Geometry: final body of the model. Coordinates: model frame, mm. Give positions to 0.01 mm unless a question says otherwise; leave off trailing zeros. Write each loop counter-clockwise with the first axis right and the second up, starting at its lowest first coordinate (ties: lowest second). Pieces come first, ordered by that corner, then holes.
from build123d import *

# Parameters (mm, degrees)
SKIZZE1_W                       = 75
SKIZZE1_H                       = 75
AUFSATZ_LINEAR_AUSTRAGEN1_DEPTH = 3
SKIZZE2_R                       = 14.5
SCHNITT_LINEAR_AUSTRAGEN1_DEPTH = 4
VERRUNDUNG1_R                   = 2
DURCHGANGSLOCH_F_R_M41_D        = 4.5
SCHNITT_LINEAR_AUSTRAGEN2_DEPTH = 4


with BuildPart() as part:
    # Skizze1 → Aufsatz-Linear austragen1 (new body)
    with BuildSketch(Plane.XY):
        Rectangle(SKIZZE1_W, SKIZZE1_H)
    extrude(amount=AUFSATZ_LINEAR_AUSTRAGEN1_DEPTH)

    # Skizze2 → Schnitt-Linear austragen1 (cut, through all)
    with BuildSketch(Plane.XY.offset(3)):
        with Locations((-18, 0)):
            Circle(SKIZZE2_R)
        with Locations((18, 0)):
            Circle(SKIZZE2_R)
    extrude(amount=-SCHNITT_LINEAR_AUSTRAGEN1_DEPTH, mode=Mode.SUBTRACT)

    # Verrundung1
    verrundung1_edges = [part.edges().sort_by_distance(p)[0] for p in [
        (37.5, -37.5, 1.5),
        (-37.5, -37.5, 1.5),
        (-37.5, 37.5, 1.5),
        (37.5, 37.5, 1.5),
    ]]
    fillet(verrundung1_edges, radius=VERRUNDUNG1_R)

    # Durchgangsloch für M41 (through all)
    with Locations(Plane.XY.offset(3)):
        with Locations((27.5, 27.5), (-27.5, 27.5)):
            durchgangsloch_f_r_m41 = Hole(DURCHGANGSLOCH_F_R_M41_D / 2)

    # Spiegeln1: Durchgangsloch für M41 across plane
    add(durchgangsloch_f_r_m41.mirror(Plane.ZX), mode=Mode.SUBTRACT)

    # Skizze6 → Schnitt-Linear austragen2 (cut, through all)
    with BuildSketch(Plane.XY.offset(3)):
        with BuildLine():
            Line((17.791240349, 1.485402103), (33.635529448, 3.712171718))
            ThreePointArc((33.635529448, 3.712171718), (35.329691203, 2.435529267), (34.053048751, 0.741367512))
            Line((34.053048751, 0.741367512), (18.208759651, -1.485402103))
            ThreePointArc((18.208759651, -1.485402103), (16.514597897, -0.208759651), (17.791240349, 1.485402103))
        make_face()
    extrude(amount=-SCHNITT_LINEAR_AUSTRAGEN2_DEPTH, mode=Mode.SUBTRACT)


solid = part.part
Q1. Pin query (flat end, axial travel): P1, Ø3.5, axis at x = 27.5, y = -27.5, coming from the -Z side. Return the tip coordinate at first contact, or that it passes through.
Filled sheet:
P1: passes through
Q2. Section C-C on z = 1.6. Output: boundary loops of the cut face in (x, y), plus the area to 3 significant figures.
Filled sheet:
outline: (-37.5, -35.5) arc R2 ccw to (-35.5, -37.5) - (35.5, -37.5) arc R2 ccw to (37.5, -35.5) - (37.5, 35.5) arc R2 ccw to (35.5, 37.5) - (-35.5, 37.5) arc R2 ccw to (-37.5, 35.5) - close; hole circle Ø29 at (-18, 0); hole circle Ø4.5 at (-27.5, -27.5); hole circle Ø4.5 at (-27.5, 27.5); hole circle Ø4.5 at (27.5, -27.5); hole circle Ø4.5 at (27.5, 27.5); hole (32.07, 3.49) arc R14.5 ccw (long way) to (32.49, 0.52) - (34.05, 0.74) arc R1.5 ccw to (33.64, 3.71) - close
area: 4,230 mm2
Q3. Section B-B on y = 27.5. Output: boundary loops of the cut face in (x, z).
Filled sheet:
outline: (-37.5, 0) - (-29.75, 0) - (-29.75, 3) - (-37.5, 3) - close; (-25.25, 0) - (25.25, 0) - (25.25, 3) - (-25.25, 3) - close; (29.75, 0) - (37.5, 0) - (37.5, 3) - (29.75, 3) - close
Q4. Pull-direction query (Y, two-part tool) for faces 1 (the flat face through (-1, 1, 0)), 2 (the cylindrical face through (-28.538, 25.504, 1.479)), 3 (the cylindrical face through (-36.93, 36.9, 1.52)); classes: released by +Y, released by -Y, zero draft, split by the parting line, or undercut.
Filled sheet:
face 1: zero draft
face 2: undercut
face 3: released by +Y
Q5. Ray query, line 1 along X through (y, z) = (1, 1.85); line 2 along Y through (x, z) = (26.5, 1.8); line 3 along Y through (x, z) = (-26, 2.3). Return the intervals inside material, ascending.
Filled sheet:
line 1: x = -37.5 to -32.47, -3.53 to 3.53, 34.71 to 37.5
line 2: y = -37.5 to -29.52, -25.48 to -11.75, 11.75 to 25.48, 29.52 to 37.5
line 3: y = -37.5 to -29.18, -25.82 to -12.09, 12.09 to 25.82, 29.18 to 37.5
Q6. Section D-D on x = 26.5. Output: boundary loops of the cut face in (y, z), plus the area to 3 significant figures.
Filled sheet:
outline: (-37.5, 0) - (-29.52, 0) - (-29.52, 3) - (-37.5, 3) - close; (-25.48, 0) - (-11.75, 0) - (-11.75, 3) - (-25.48, 3) - close; (11.75, 0) - (25.48, 0) - (25.48, 3) - (11.75, 3) - close; (29.52, 0) - (37.5, 0) - (37.5, 3) - (29.52, 3) - close
area: 130 mm2
Q7. Section A-A on x = -18. Output: boundary loops of the cut face in (y, z), plus the area to 3 significant figures.
Filled sheet:
outline: (-37.5, 0) - (-14.5, 0) - (-14.5, 3) - (-37.5, 3) - close; (14.5, 0) - (37.5, 0) - (37.5, 3) - (14.5, 3) - close
area: 138 mm2
